Design review of the part built by this model. Coordinates are the model's own, in mm. Face numbers are marked on the shaded views. A direction names the side the tool comes from. Round coordinates to 2 decimals unless told otherwise and drop trailing zeros. Order: outer loops, then holes, each group sorted by start corner. A loop starts at its lowest first (then second) coordinate and runs counter-clockwise, first axis right, second up. Notation, with made-up numbers: M 67,-34 L 84,-34 A17 ccw 84,-26 Z; hole C 50.5,29.5 d3. An arc over 180 degrees is marked long. Use a Markdown table: item, result. Add a question column.
(1) Take a section at A-A (x = 26). Write out the cut boundary in (y, z), then the cut area to 3 significant figures.
(2) The part is to be moulded in two halves that separate along X. For the marked faces 3, 4 and 5, say which applies: released by +X, released by -X, zero draft, split by the parting line, or undercut.
(3) To check wall thickness, follow probe 1 along Z at (x, y) = (7, 60.5); probe 2 along X at (y, z) = (10, 0). State the ranges of each line that lie inside material, in increasing order. Write a range as from..to.
(4) Take a section at C-C (y = 13). Write out the cut boundary in (x, z), then the cut area to 3 significant figures.
(5) For pin 1 (1.4 mm diameter, centred on x = 51, z = 0.5, fed in from -Y); pin 2 (2.5 mm diameter, centred on x = -0.5, z = -47, fed in from +Y); pin 3 (16.5 mm diameter, centred on x = 6, y = 50, fed in from -Z); pin 4 (4 mm diameter, centred on x = -18.5, y = 36.5, fed in from +Z), all flat-tipped, find the tip position at first contact; note any pin that passes through.
(6) Take a section at B-B (z = -3.5). Write out the cut boundary in (x, y), then the cut area to 3 significant figures.
(7) Machinability: for the marked faces 1 and 2, which of the approach directions +Z, -Z, +X, -X, +Y, -Y give a long, thin tool a straight path to every point of the face, cutting with its end or side? Answer none if there is none.
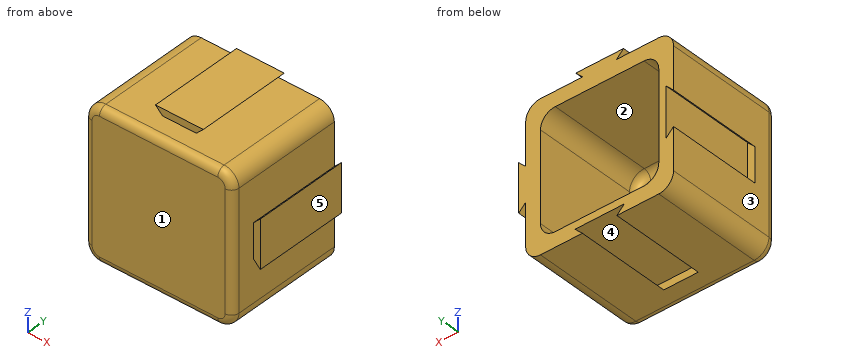
```python
from build123d import *

# Parameters (mm, degrees)
SKETCH1_W                 = 100
SKETCH1_H                 = 100
BOSS_EXTRUDE1_DEPTH       = 80
SHELL1_T                  = -10
SHELL1_THICKNESS_2_FACE_W = 80
SHELL1_THICKNESS_2_FACE_H = 80
SHELL1_THICKNESS_2_DEPTH  = 5
CUT_EXTRUDE1_DEPTH        = 64
BOSS_EXTRUDE2_DEPTH       = 63.7
CUT_EXTRUDE2_DEPTH        = 64
BOSS_EXTRUDE3_DEPTH       = 63.7
FILLET1_R                 = 10
FILLET2_R                 = 5


with BuildPart() as part:
    # Sketch1 → Boss-Extrude1 (new body)
    with BuildSketch(Plane(origin=(0, 0, 0), x_dir=(1, 0, 0), z_dir=(0, 1, 0))):
        Rectangle(SKETCH1_W, SKETCH1_H)
    extrude(amount=BOSS_EXTRUDE1_DEPTH)

    # Shell1
    shell1_openings = [part.faces().sort_by_distance(p)[0] for p in [
        (0, 80, 0),
    ]]
    offset(amount=SHELL1_T, openings=shell1_openings, kind=Kind.INTERSECTION)

    # Shell1 thickness 2 face (on inner face of the shell) → Shell1 thickness 2 (cut)
    with BuildSketch(Plane(origin=(0, 10, 0), x_dir=(0, 0, -1), z_dir=(0, -1, 0))):
        Rectangle(SHELL1_THICKNESS_2_FACE_W, SHELL1_THICKNESS_2_FACE_H)
    extrude(amount=SHELL1_THICKNESS_2_DEPTH, mode=Mode.SUBTRACT)

    # Sketch2 → Cut-Extrude1 (cut)
    with BuildSketch(Plane(origin=(0, 80, 0), x_dir=(1, 0, 0), z_dir=(0, 1, 0))):
        Polygon((-11.666666667, 50), (-16.666666667, 45), (16.666666667, 45), (11.666666667, 50), align=None)
    extrude(amount=-CUT_EXTRUDE1_DEPTH, mode=Mode.SUBTRACT)

    # Sketch3 → Boss-Extrude2 (add)
    with BuildSketch(Plane(origin=(0, 80, 0), x_dir=(1, 0, 0), z_dir=(0, 1, 0))):
        Polygon((-11.454534632, -50), (-16.154534632, -54.7), (16.154534632, -54.7), (11.454534632, -50), align=None)
    extrude(amount=-BOSS_EXTRUDE2_DEPTH)

    # Sketch4 → Cut-Extrude2 (cut)
    with BuildSketch(Plane(origin=(0, 80, 0), x_dir=(1, 0, 0), z_dir=(0, 1, 0))):
        Polygon((-45, 16.666666667), (-45, -16.666666667), (-50, -11.666666667), (-50, 11.666666667), align=None)
    extrude(amount=-CUT_EXTRUDE2_DEPTH, mode=Mode.SUBTRACT)

    # Sketch5 → Boss-Extrude3 (add)
    with BuildSketch(Plane(origin=(0, 80, 0), x_dir=(1, 0, 0), z_dir=(0, 1, 0))):
        Polygon((50, 11.454534632), (50, -11.454534632), (54.7, -16.154534632), (54.7, 16.154534632), align=None)
    extrude(amount=-BOSS_EXTRUDE3_DEPTH)

    # Fillet1
    fillet1_edges = [part.edges().sort_by_distance(p)[0] for p in [
        (40, 42.5, 40),
        (40, 42.5, -40),
        (-40, 42.5, -40),
        (-40, 42.5, 40),
        (50, 40, 50),
        (-50, 40, 50),
        (-50, 40, -50),
        (50, 40, -50),
    ]]
    fillet(fillet1_edges, radius=FILLET1_R)

    # Fillet2
    fillet2_edges = [part.edges().sort_by_distance(p)[0] for p in [
        (50, 0, 0),
        (0, 0, 50),
        (-50, 0, 0),
        (47.071067812, 0, 47.071067812),
        (-47.071067812, 0, 47.071067812),
        (-47.071067812, 0, -47.071067812),
        (47.071067812, 0, -47.071067812),
        (40, 5, 0),
        (0, 5, -40),
        (-40, 5, 0),
        (0, 5, 40),
        (37.071067812, 5, 37.071067812),
        (-37.071067812, 5, 37.071067812),
        (-37.071067812, 5, -37.071067812),
        (37.071067812, 5, -37.071067812),
        (0, 0, -50),
    ]]
    fillet(fillet2_edges, radius=FILLET2_R)


solid = part.part
```
Verdict:
| question | item | result |
|---|---|---|
| 1 | outline | M 0,-45 A5 ccw 5,-50 L 80,-50 L 80,-40 L 10,-40 A5 cw 5,-35 L 5,35 A5 cw 10,40 L 80,40 L 80,50 L 5,50 A5 ccw 0,45 Z |
| 1 | area | 2,000 mm^2 |
| 2 | face 3 | released by -X |
| 2 | face 4 | undercut |
| 2 | face 5 | released by +X |
| 3 | probe 1 | z = -45..-40, 40..54.7 |
| 3 | probe 2 | x = -50..-40, 40..50 |
| 4 | outline | M -50,-40 A10 ccw -40,-50 L 40,-50 A10 ccw 50,-40 L 50,40 A10 ccw 40,50 L -40,50 A10 ccw -50,40 Z; hole M -40,-30 A10 ccw -30,-40 L 30,-40 A10 ccw 40,-30 L 40,30 A10 ccw 30,40 L -30,40 A10 ccw -40,30 Z |
| 4 | area | 3,600 mm^2 |
| 5 | pin 1 | stops at y = 16.3 |
| 5 | pin 2 | stops at y = 16 |
| 5 | pin 3 | stops at z = -50 |
| 5 | pin 4 | stops at z = 50 |
| 6 | outline | M -50,5 A5 ccw -45,0 L 45,0 A5 ccw 50,5 L 50,16.3 L 54.7,16.3 L 54.7,80 L 40,80 L 40,10 A5 cw 35,5 L -35,5 A5 cw -40,10 L -40,80 L -45,80 L -45,16 L -50,16 Z |
| 6 | area | 1,980 mm^2 |
| 7 | face 1 | +Z, -Z, +X, -X, -Y |
| 7 | face 2 | +Y |
